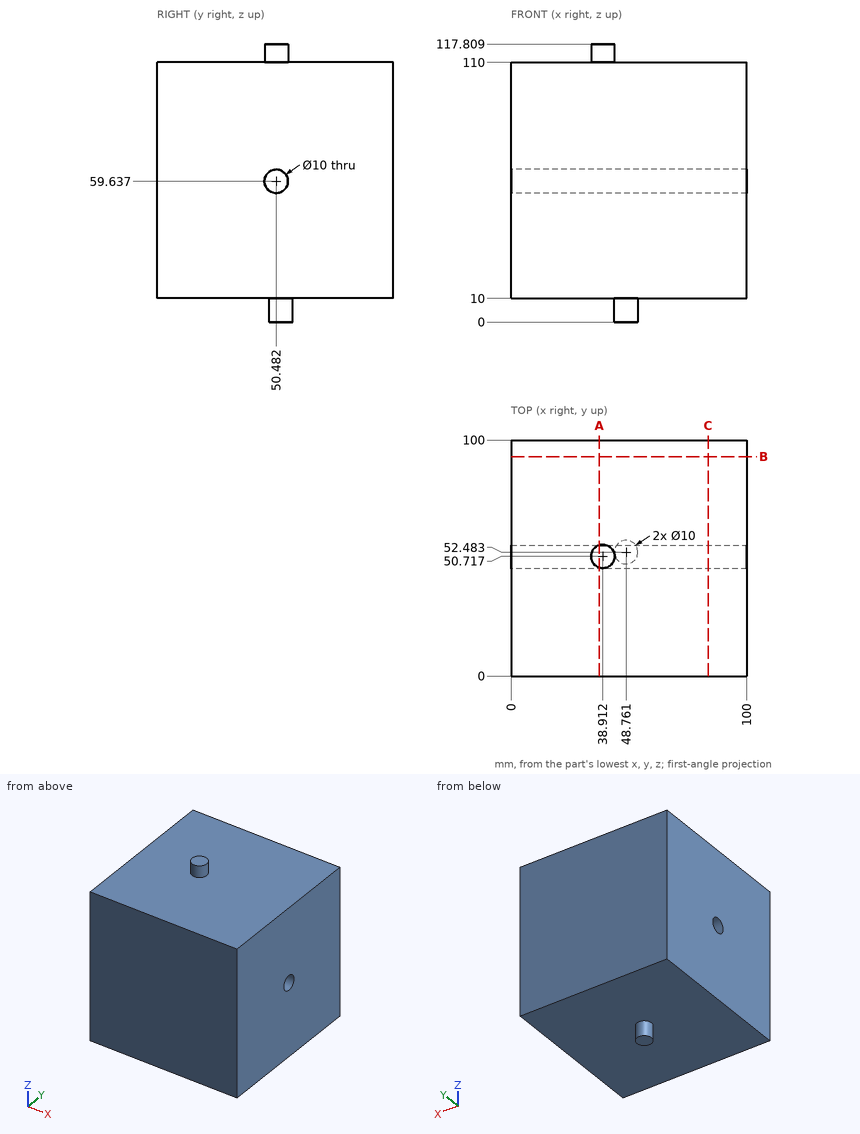
Source: three-view drawing plus pictorial views. Frame: mm from the lowest corner of the part. Coordinates: 2 decimals unless noted, no trailing zeros. Order: outer loops, then holes, each group sorted by start corner. A loop starts at its lowest first (then second) coordinate and runs counter-clockwise, first axis right, second up. Notation, with made-up numbers: M 27,75 L 80,75 A27 cw 80,106 Z; hole C 45,-22.5 d2. An arc over 180 degrees is marked long. One line per question, with ' | ' between items. Start each with the question number.
Item 1: Cut plane A-A, the plane x = 37.5. Return the cut outline in (y, z).
Item 2: Cut plane B-B, the plane y = 93. Return the cut outline in (x, z), then the cut area to 3 significant figures.
Item 3: Ray query, probe 1 along Z at (x, y) = (80, 86); probe 2 along Y at (x, z) = (78.5, 59); probe 3 along Z at (x, y) = (15.5, 49). Return the intervals inside material, ascending. Write a range as [from, to].
Item 4: Cut plane C-C, the plane x = 83.5. Return the cut outline in (y, z), then the cut area to 3 significant figures.
Item 5: Pin query (flat end, axial travel): pin 1 Ø5 at (x, y) = (63.5, 43.5) entering from +Z; pin 2 Ø5 at (x, y) = (39, 78.5) entering from -Z. Return the tip coordinate at first contact, or that it passes through.
A:
1) outline: M 0,10 L 100,10 L 100,110 L 55.51,110 L 55.51,117.81 L 45.92,117.81 L 45.92,110 L 0,110 Z; hole C 50.48,59.64 d10
2) outline: M 0,10 L 100,10 L 100,110 L 0,110 Z | area: 10,000 mm2
3) probe 1: z = [10, 110] | probe 2: y = [0, 45.52], [55.44, 100] | probe 3: z = [10, 54.86], [64.41, 110]
4) outline: M 0,10 L 100,10 L 100,110 L 0,110 Z; hole C 50.48,59.64 d10 | area: 9,920 mm2
5) pin 1: stops at z = 110 | pin 2: stops at z = 10
